Verification items for this drawing (mm, ordinates from the low corner). Round coordinates to 2 decimals unless told otherwise and drop trailing zeros. Order: outer loops, then holes, each group sorted by start corner. A loop starts at its lowest first (then second) coordinate and runs counter-clockwise, first axis right, second up. Notation, with made-up numbers: (7, 40) -> (20, 40) arc R17 cw to (20, 46) -> close; hole circle Ø10 at (39.25, 67.25). An arc over 180 degrees is marked (long way). Answer in a Markdown table with one row per item. Add a question column.
1. Draft check along X on the marked faces 1, 2 and 3. Enter one of: +X half, -X half, draft (parallel to the pull), parting line (faces both ways), or undercut.
2. Sectioned sample at A-A, the plane x = 9.5. Record the boundary of the cut face in (y, z), then the cut area to 3 significant figures.
3. Sectioned sample at C-C, the plane z = 1. Record the boundary of the cut face in (x, y).
4. Depth check by flat-ended pin: P1, Ø1, axis at y = 15, z = 3, coming from the -X side; P2, Ø1, axis at y = 14, z = 3.5, coming from the +X side; P3, Ø1, axis at y = 3, z = 6.5, coming from the +X side. Enter the tip coordinate at first touch or a pass-through.
5. Sectioned sample at D-D, the plane y = 3.25. Record the boundary of the cut face in (x, z).
6. Material ranges on L1, parallel to Y at x = 9.5, z = 5.75; L2, parallel to Z at x = 17.5, y = 8; L3, parallel to X at y = 7.75, z = 7.5, recorded low to high. Write a range as from..to.
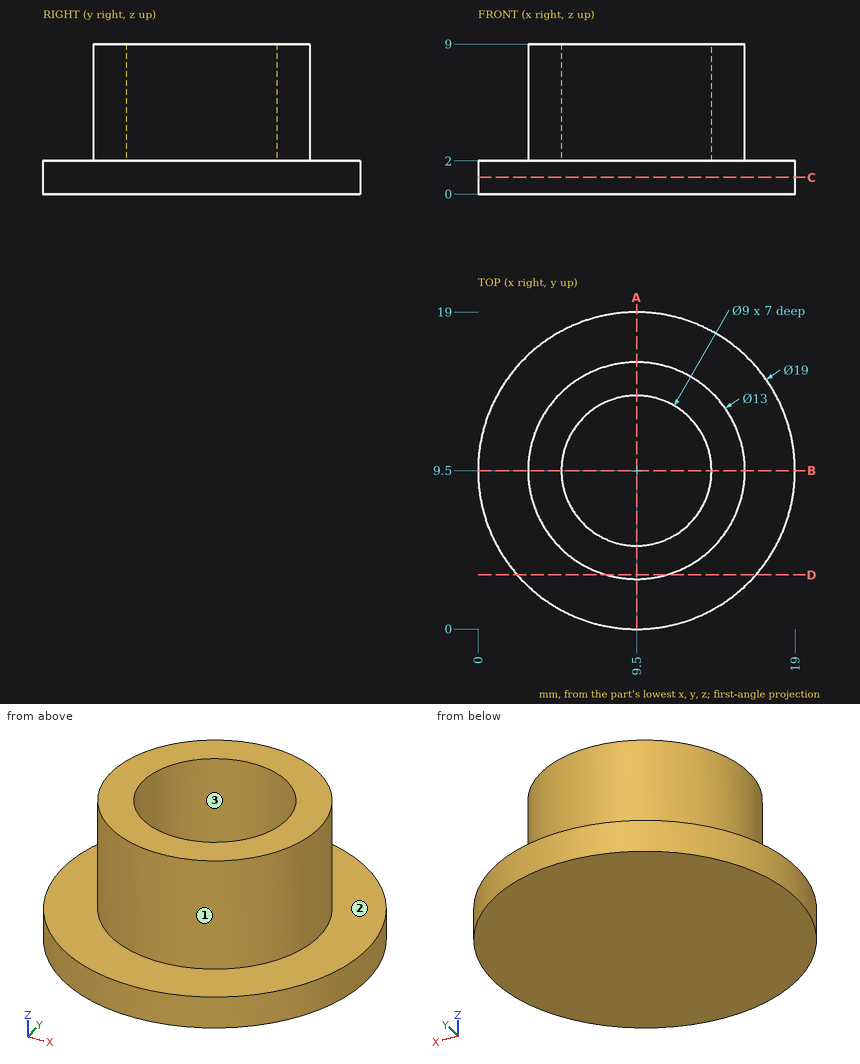
Answer key:
| question | item | result |
|---|---|---|
| 1 | face 1 | parting line |
| 1 | face 2 | draft |
| 1 | face 3 | undercut |
| 2 | outline | (0, 0) -> (19, 0) -> (19, 2) -> (16, 2) -> (16, 9) -> (14, 9) -> (14, 2) -> (5, 2) -> (5, 9) -> (3, 9) -> (3, 2) -> (0, 2) -> close |
| 2 | area | 66.0 mm² |
| 3 | outline | circle Ø19 at (9.5, 9.5) |
| 4 | P1 | stops at x = 5.35 |
| 4 | P2 | stops at x = 14.62 |
| 4 | P3 | stops at x = 12 |
| 5 | outline | (2.35, 0) -> (16.65, 0) -> (16.65, 2) -> (11.29, 2) -> (11.29, 9) -> (7.71, 9) -> (7.71, 2) -> (2.35, 2) -> close |
| 6 | L1 | y = 3..5, 14..16 |
| 6 | L2 | z = 0..2 |
| 6 | L3 | x = 3.24..5.35, 13.65..15.76 |
